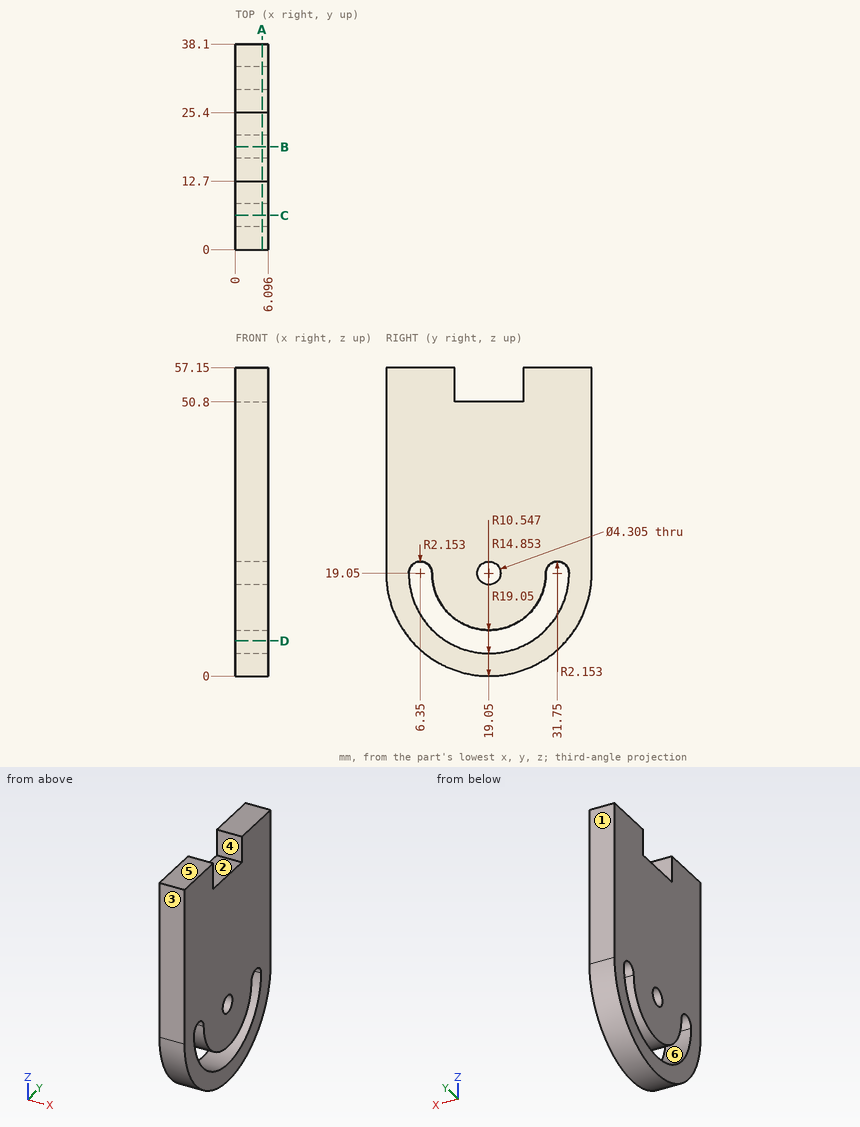
Answer from the drawing. Dimensions are ordinates in mm from the lowest x, y and z of the part. A direction names the side the tool comes from. Round coordinates to 2 decimals unless told otherwise and drop trailing zeros. Loops run counter-clockwise (first coordinate to the right, second up) from the corner with the lowest first, then second, coordinate; pieces in that order, holes last.
1) A cutting plane is placed at B-B on y = 19.05. Determine the outline of the cut face in (x, z), plus the area to 3 significant figures.
Outcome:
outline: (0, 0) - (6.1, 0) - (6.1, 4.2) - (0, 4.2) - close; (0, 8.5) - (6.1, 8.5) - (6.1, 16.9) - (0, 16.9) - close; (0, 21.2) - (6.1, 21.2) - (6.1, 50.8) - (0, 50.8) - close
area: 257 mm2
2) For the marked faces 4, 5 and 6, determine the directions among +Z, -Z, +X, -X, +Y, -Y from which every point of the face is accessible in a straight line to the end or side of a thin tool.
Outcome:
face 4: +Z, +X, -X
face 5: +Z, +X, -X, +Y, -Y
face 6: +X, -X
3) Given P1, Ø1.8, axis at x = 3.5, y = 17.5, coming from the +Z side, flat-ended and moving along its own axis, determine where the tip first touches the part or whether it passes through.
Outcome:
P1: stops at z = 50.8
4) A cutting plane is placed at A-A on x = 5. Give the number of separate pieces and of enclosed holes in the cut face, plus the area to 3 significant figures.
Outcome:
separate pieces: 1
enclosed holes: 2
area: 1,740 mm2
5) A cutting plane is placed at D-D on z = 6.5. Determine the outline of the cut face in (x, y).
Outcome:
outline: (0, 4.72) - (6.1, 4.72) - (6.1, 11.11) - (0, 11.11) - close; (0, 26.99) - (6.1, 26.99) - (6.1, 33.38) - (0, 33.38) - close
6) A cutting plane is placed at C-C on y = 6.35. Determine the outline of the cut face in (x, z).
Outcome:
outline: (0, 4.85) - (6.1, 4.85) - (6.1, 11.35) - (0, 11.35) - close; (0, 21.2) - (6.1, 21.2) - (6.1, 57.15) - (0, 57.15) - close
7) Consider line 1 (Y direction, x = 3, z = 19.05); line 2 (Y direction, x = 4.25, z = 51); line 3 (Z direction, x = 3.5, y = 20.5) (1 decimal). Determine where each line is inside the solid, lowest interval first.
Outcome:
line 1: y = 0 to 4.2, 8.5 to 16.9, 21.2 to 29.6, 33.9 to 38.1
line 2: y = 0 to 12.7, 25.4 to 38.1
line 3: z = 0.1 to 4.3, 8.6 to 17.5, 20.6 to 50.8
8) For a pull along Y with two mould halves and no side action, classify the marked faces 1, 2 and 3 as released by +Y, released by -Y, zero draft, split by the parting line, or undercut.
Outcome:
face 1: released by +Y
face 2: undercut
face 3: released by -Y
